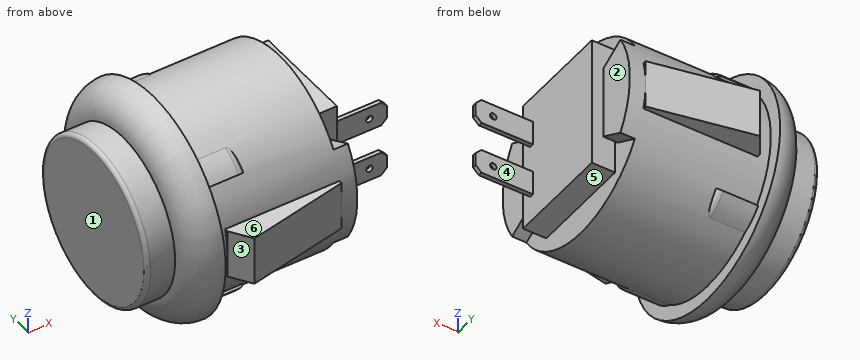
from build123d import *

# Parameters (mm, degrees)
BOSS_EXTRUDE4_START = 5.26
BOSS_EXTRUDE4_DEPTH = 5.26
FILLET2_R           = 1
SKETCH8_OUTSIDE_W   = 38.012
SKETCH8_OUTSIDE_H   = 38.012
CUT_EXTRUDE2_DEPTH  = 1.77
BOSS_EXTRUDE1_DEPTH = 2.85
SKETCH3_W           = 3.0000000000000004
SKETCH3_H           = 0.5
SKETCH3_W_2         = 3.000000000000001
BOSS_EXTRUDE2_DEPTH = 7
SKETCH4_R           = 0.40000000000000124
CUT_EXTRUDE1_DEPTH  = 40.59712936066199
CHAMFER1_SIZE       = 0.7
BOSS_EXTRUDE3_DEPTH = 3
FILLET1_R           = 0.5


with BuildPart() as part:
    # Sketch1 → Revolve1 (revolve)
    with BuildSketch(Plane.XY, mode=Mode.PRIVATE) as revolve1_sk:
        with BuildLine():
            Line((0, 0), (0, 9.75))
            Line((0, 9.75), (3.4999999999999996, 9.749999999999998))
            ThreePointArc((3.4999999999999996, 9.749999999999998), (4.591027240080107, 12.383972759919889), (7.224999999999997, 13.474999999999998))
            Line((7.224999999999997, 13.474999999999998), (7.224999999999998, 11.75))
            Line((7.224999999999998, 11.75), (24.5, 11.75))
            Line((24.5, 11.75), (24.5, 0))
            Line((24.5, 0), (0, 0))
        make_face()
    revolve(revolve1_sk.sketch.rotate(Axis((24.5, 0, 0), (-1, 0, 0)), 90), axis=Axis((24.5, 0, 0), (-1, 0, 0)))

    # Sketch7 → Boss-Extrude4 (add)
    with BuildSketch(Plane(origin=(7.224999999999997, 0, 0), x_dir=(0, 0, -1), z_dir=(1, 0, 0)).offset(BOSS_EXTRUDE4_START)):
        with BuildLine():
            Line((-7.337277205884233, 9.177519447215122), (-7.540223171153369, 9.431365729797664))
            ThreePointArc((-7.540223171153369, 9.431365729797664), (-8.631515815707116, 8.327069376529131), (-9.437293044088438, 7))
            ThreePointArc((-9.437293044088438, 7), (-8.457656265394512, 8.156626171183342), (-7.337277205884233, 9.177519447215122))
        make_face()
        with BuildLine():
            Line((-7.337277205884229, -9.177519447215122), (-7.540223171153365, -9.431365729797664))
            ThreePointArc((-7.540223171153365, -9.431365729797664), (-8.631515815707113, -8.327069376529131), (-9.437293044088431, -7))
            ThreePointArc((-9.437293044088431, -7), (-8.457656265394512, -8.15662617118334), (-7.337277205884229, -9.177519447215122))
        make_face()
        with BuildLine():
            Line((7.337277205884229, -9.177519447215122), (7.540223171153365, -9.431365729797664))
            ThreePointArc((7.540223171153365, -9.431365729797664), (8.631515815707113, -8.327069376529131), (9.437293044088431, -7))
            ThreePointArc((9.437293044088431, -7), (8.45765626539451, -8.156626171183342), (7.337277205884229, -9.177519447215122))
        make_face()
        with BuildLine():
            Line((7.337277205884233, 9.177519447215122), (7.540223171153369, 9.431365729797664))
            ThreePointArc((7.540223171153369, 9.431365729797664), (8.631515815707118, 8.32706937652913), (9.437293044088438, 7))
            ThreePointArc((9.437293044088438, 7), (8.457656265394514, 8.15662617118334), (7.337277205884233, 9.177519447215122))
        make_face()
    extrude(amount=-BOSS_EXTRUDE4_DEPTH)

    # Fillet2
    # the kernel refuses this fillet: 1 mm, written as the material it takes off along each edge
    with BuildSketch(Plane(origin=(12.484999999999996, -4.232653152686616, 3.383937203973504), x_dir=(0, -0.9556882368173963, 0.2943806957136558), z_dir=(0, -0.2943806957136558, -0.9556882368173963))) as fillet2_piece_1_section:
        with BuildLine():
            CenterArc((6.655924090642022 - FILLET2_R, FILLET2_R), FILLET2_R, 270, 90)
            Line((6.655924090642022 - FILLET2_R, 0), (6.655924090642022, 0))
            Line((6.655924090642022, 0), (6.6559240906420225, FILLET2_R))
        make_face()
    fillet2_piece_1 = revolve(axis=Axis((12.484999999999996, -4.232653152686616, 3.383937203973504), (-1, 0, 0)), revolution_arc=69.83301403972071, mode=Mode.PRIVATE)
    fillet2_piece_1 = fillet2_piece_1 - Plane(origin=(12.185339920044097, 0, 0), x_dir=(0, 1.1e-16, -1), z_dir=(1, 0, 0)) * Cylinder(11.75, 27, mode=Mode.PRIVATE)
    add(fillet2_piece_1, mode=Mode.SUBTRACT)
    with BuildSketch(Plane(origin=(12.484999999999996, -4.232653152686616, -3.383937203973504), x_dir=(0, -0.9556882368173963, -0.2943806957136558), z_dir=(0, -0.2943806957136558, 0.9556882368173963))) as fillet2_piece_2_section:
        with BuildLine():
            CenterArc((6.655924090642022 - FILLET2_R, -FILLET2_R), FILLET2_R, 0, 90)
            Line((6.655924090642022 - FILLET2_R, 0), (6.655924090642022, 0))
            Line((6.655924090642022, 0), (6.6559240906420225, -FILLET2_R))
        make_face()
    fillet2_piece_2 = revolve(axis=Axis((12.484999999999996, -4.232653152686616, -3.383937203973504), (1, 0, 0)), revolution_arc=69.83301403972071, mode=Mode.PRIVATE)
    fillet2_piece_2 = fillet2_piece_2 - Plane(origin=(12.185339900483468, 0, 0), x_dir=(0, 1.1e-16, -1), z_dir=(1, 0, 0)) * Cylinder(11.75, 27, mode=Mode.PRIVATE)
    add(fillet2_piece_2, mode=Mode.SUBTRACT)
    with BuildSketch(Plane(origin=(12.484999999999996, 4.2326531526865825, -3.383937203973474), x_dir=(0, 0.9556882368173955, -0.29438069571365894), z_dir=(0, 0.29438069571365894, 0.9556882368173955))) as fillet2_piece_3_section:
        with BuildLine():
            CenterArc((6.65592409064207 - FILLET2_R, FILLET2_R), FILLET2_R, 270, 90)
            Line((6.65592409064207 - FILLET2_R, 0), (6.65592409064207, 0))
            Line((6.65592409064207, 0), (6.65592409064207, FILLET2_R))
        make_face()
    fillet2_piece_3 = revolve(axis=Axis((12.484999999999996, 4.2326531526865825, -3.383937203973474), (-1, 0, 0)), revolution_arc=69.83301403972023, mode=Mode.PRIVATE)
    fillet2_piece_3 = fillet2_piece_3 - Plane(origin=(12.185339920045562, 0, 0), x_dir=(0, 1.1e-16, -1), z_dir=(1, 0, 0)) * Cylinder(11.75, 27, mode=Mode.PRIVATE)
    add(fillet2_piece_3, mode=Mode.SUBTRACT)
    with BuildSketch(Plane(origin=(12.484999999999996, 4.232653152686593, 3.3839372039734887), x_dir=(0, 0.955688236817396, 0.29438069571365705), z_dir=(0, 0.29438069571365705, -0.955688236817396))) as fillet2_piece_4_section:
        with BuildLine():
            CenterArc((6.65592409064205 - FILLET2_R, -FILLET2_R), FILLET2_R, 0, 89.99999999999994)
            Line((6.65592409064205 - FILLET2_R, 0), (6.65592409064205, 0))
            Line((6.65592409064205, 0), (6.655924090642049, -FILLET2_R))
        make_face()
    fillet2_piece_4 = revolve(axis=Axis((12.484999999999996, 4.232653152686593, 3.3839372039734887), (1, 0, 0)), revolution_arc=69.83301403972044, mode=Mode.PRIVATE)
    fillet2_piece_4 = fillet2_piece_4 - Plane(origin=(12.185339900321193, 0, 0), x_dir=(0, 1.1e-16, -1), z_dir=(1, 0, 0)) * Cylinder(11.75, 27, mode=Mode.PRIVATE)
    add(fillet2_piece_4, mode=Mode.SUBTRACT)

    # Sketch8 outside → Cut-Extrude2 (cut)
    with BuildSketch(Plane(origin=(24.5, 0, 0), x_dir=(0, 0, -1), z_dir=(1, 0, 0))):
        Rectangle(SKETCH8_OUTSIDE_W, SKETCH8_OUTSIDE_H)
        with BuildLine():
            Line((-6.1499999999999995, 10.011992808627065), (-4.5, 6.85))
            Line((-4.5, 6.85), (4.5, 6.85))
            Line((4.5, 6.85), (6.1499999999999995, 10.011992808627065))
            ThreePointArc((6.1499999999999995, 10.011992808627065), (7.2e-16, 11.750000000000002), (-6.1499999999999995, 10.011992808627065))
        make_face(mode=Mode.SUBTRACT)
        with BuildLine():
            Line((4.5, -6.85), (6.1499999999999995, -10.011992808627065))
            ThreePointArc((6.1499999999999995, -10.011992808627065), (7.2e-16, -11.750000000000002), (-6.1499999999999995, -10.011992808627065))
            Line((-6.1499999999999995, -10.011992808627065), (-4.5, -6.85))
            Line((-4.5, -6.85), (4.5, -6.85))
        make_face(mode=Mode.SUBTRACT)
    extrude(amount=-CUT_EXTRUDE2_DEPTH, mode=Mode.SUBTRACT)

    # Sketch2 → Boss-Extrude1 (add)
    with BuildSketch(Plane(origin=(22.73, 0, 0), x_dir=(0, 0, -1), z_dir=(1, 0, 0))):
        Polygon((-8.100000000000001, 6.35), (8.099999999999998, 6.35), (8.1, -6.35), (-8.1, -6.35), align=None)
    extrude(amount=BOSS_EXTRUDE1_DEPTH)

    # Sketch3 → Boss-Extrude2 (add)
    with BuildSketch(Plane(origin=(25.58, 0, 0), x_dir=(0, 0, -1), z_dir=(1, 0, 0))):
        with Locations((-3.3, -4.8)):
            Rectangle(SKETCH3_W, SKETCH3_H)
        with Locations((3.300000000000001, -4.799999999999999)):
            Rectangle(SKETCH3_W_2, SKETCH3_H)
    extrude(amount=BOSS_EXTRUDE2_DEPTH)

    # Sketch4 → Cut-Extrude1 (cut, through all)
    with BuildSketch(Plane(origin=(0, -4.55, 0), x_dir=(-1, 0, 0), z_dir=(0, 1, -6e-17))):
        with Locations(Location((-30.43, 3.2999999999999994, 0), (0, 0, 90))):
            Circle(SKETCH4_R)
        with Locations(Location((-30.43, -3.3000000000000007, 0), (0, 0, 90))):
            Circle(SKETCH4_R)
    extrude(amount=-CUT_EXTRUDE1_DEPTH, mode=Mode.SUBTRACT)

    # Chamfer1
    chamfer1_edges = [part.edges().sort_by_distance(p)[0] for p in [
        (32.58, -4.8, 1.7999999999999996),
        (32.58, -4.8, 4.8),
        (32.58, -4.799999999999999, -4.800000000000002),
        (32.58, -4.799999999999999, -1.8000000000000007),
    ]]
    chamfer(chamfer1_edges, length=CHAMFER1_SIZE)

    # Sketch5 → Boss-Extrude3 (add, symmetric)
    with BuildSketch(Plane.XY):
        Polygon((22.56668760482229, -11.75), (10.224999999999994, -14.25), (8.566687604822294, -11.750000000000002), (8.566687604822294, -10.750000000000002), (22.56668760482229, -10.75), align=None)
        Polygon((8.56668760482229, 10.750000000000005), (8.56668760482229, 11.750000000000005), (10.22499999999999, 14.250000000000004), (22.566687604822288, 11.750000000000007), (22.566687604822288, 10.750000000000007), align=None)
    extrude(amount=BOSS_EXTRUDE3_DEPTH, both=True)

    # Fillet1
    fillet1_edges = [part.edges().sort_by_distance(p)[0] for p in [
        (0, -2.28e-15, 9.75),
    ]]
    fillet(fillet1_edges, radius=FILLET1_R)


solid = part.part
Work out the finished part from the listing and answer in its coordinate system (mm). Face numbers are marked on the shaded views. A direction names the side the tool comes from. Give positions to 0.01 mm unless a question says otherwise; leave off trailing zeros. Loops run counter-clockwise (first coordinate to the right, second up) from the corner with the lowest first, then second, coordinate; pieces in that order, holes last. Notation, with made-up numbers: (77.25, 46) -> (123.25, 46) arc R16 cw to (123.25, 64) -> close; hole circle Ø8 at (71, 70.25). An arc over 180 degrees is marked (long way). Use a Markdown table: item, result. Add a question column.
1) The part is cut by section C-C, the plane x = 17.5. Determine the outline of the cut face in (y, z), plus the area to 3 significant figures.
2) For a pull along X with two mould halves and no side action, classify the marked faces 1, 2 and 3 as +X half, -X half, draft (parallel to the pull), parting line (faces both ways), or undercut.
3) The part is cut by section A-A, the plane y = 0. Determine the outline of the cut face in (x, z) (3 decimals), plus the area to 3 significant figures.
4) Consider line 1 along Z through (x, y) = (30.43, -4.9); line 2 along Y through (x, z) = (23.5, 3); line 3 along X through (y, z) = (-4.7, 3.3). Determine where each line is inside the solid, lowest interval first.
5) The part is cut by section B-B, the plane x = 21.5. Determine the outline of the cut face in (y, z), plus the area to 3 significant figures.
6) Which of the six approach directions +Z, -Z, +X, -X, +Y, -Y give full straight-line access (tool end or side, diameter ignored) to the marked faces 4, 5 and 6?
7) Each of these flat-tipped pins is pushed along its axis until it touches: P1, Ø3, axis at x = 24, z = 0.5, coming from the +Y side; P2, Ø0.9, axis at x = 23.5, y = 0, coming from the -Z side; P3, Ø0.9, axis at x = 16, y = -12.5, coming from the +Z side. Where does it stop, or does it pass through?
Reported:
| question | item | result |
|---|---|---|
| 1 | outline | (-12.78, -3) -> (-11.36, -3) arc R11.75 ccw to (11.36, -3) -> (12.78, -3) -> (12.78, 3) -> (11.36, 3) arc R11.75 ccw to (-11.36, 3) -> (-12.78, 3) -> close |
| 1 | area | 448 mm^2 |
| 2 | face 1 | -X half |
| 2 | face 2 | +X half |
| 2 | face 3 | undercut |
| 3 | outline | (0, -9.25) arc R0.5 ccw to (0.5, -9.75) -> (3.5, -9.75) arc R3.725 ccw to (7.225, -13.475) -> (7.225, -11.75) -> (22.73, -11.75) -> (22.73, -8.1) -> (25.58, -8.1) -> (25.58, 8.1) -> (22.73, 8.1) -> (22.73, 11.75) -> (7.225, 11.75) -> (7.225, 13.475) arc R3.725 ccw to (3.5, 9.75) -> (0.5, 9.75) arc R0.5 ccw to (0, 9.25) -> close |
| 3 | area | 573 mm^2 |
| 4 | line 1 | z = -4.8 to -3.7, -2.9 to -1.8, 1.8 to 2.9, 3.7 to 4.8 |
| 4 | line 2 | y = -11.36 to -6.85, -6.35 to 6.35, 6.85 to 11.36 |
| 4 | line 3 | x = 0 to 30.03, 30.83 to 32.58 |
| 5 | outline | (-11.97, -3) -> (-11.36, -3) arc R11.75 ccw to (11.36, -3) -> (11.97, -3) -> (11.97, 3) -> (11.36, 3) arc R11.75 ccw to (-11.36, 3) -> (-11.97, 3) -> close |
| 5 | area | 438 mm^2 |
| 6 | face 4 | +Z, -Z, +X, +Y |
| 6 | face 5 | -Z, +X, +Y, -Y |
| 6 | face 6 | +Z, +X, -Y |
| 7 | P1 | stops at y = 11.76 |
| 7 | P2 | stops at z = -8.1 |
| 7 | P3 | stops at z = 3 |
